```python
from build123d import *

# Parameters (mm, degrees)
F0_W     = 38.1
F0_H     = 38.1
F1_DEPTH = 177.8
F2_T     = -2.54
F3_R     = 2.579688
F4_DEPTH = 355.601
F5_R     = 3.175
F6_DEPTH = 38.101


with BuildPart() as f1:
    # F0 (on Front) → F1 (new body, symmetric)
    with BuildSketch(Plane.XZ):
        Rectangle(F0_W, F0_H)
    extrude(amount=F1_DEPTH, both=True)

    # F2
    f2_openings = [f1.faces().sort_by_distance(p)[0] for p in [
        (-19.05, 0, 0),
        (0, 0, -19.05),
    ]]
    offset(amount=F2_T, openings=f2_openings)

    # F3 (on face) → F4 (cut, through all)
    with BuildSketch(Plane(origin=(0, 177.8, 0), x_dir=(-1, 0, 0), z_dir=(0, 1, 0))):
        Circle(F3_R)
    extrude(amount=-F4_DEPTH, mode=Mode.SUBTRACT)

    # F5 (on face) → F6 (cut, through all)
    with BuildSketch(Plane.YZ.offset(19.05)):
        with Locations((-101.6, 0)):
            Circle(F5_R)
        with Locations((101.6, 0)):
            Circle(F5_R)
    extrude(amount=-F6_DEPTH, mode=Mode.SUBTRACT)


solid = f1.part
```
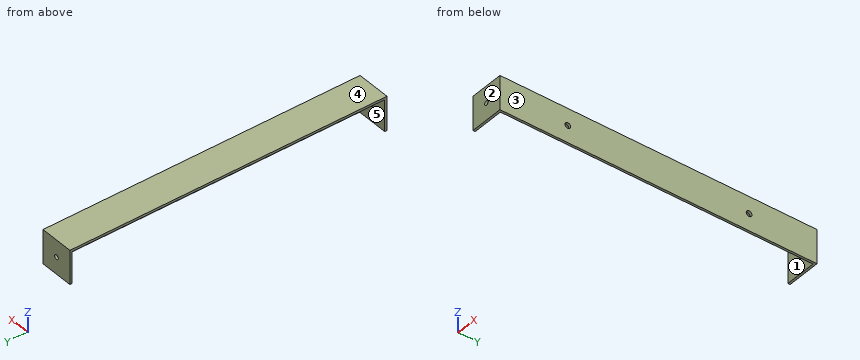
Verification items for the finished model (mm, model axes). Face numbers are marked on the shaded views. A direction names the side the tool comes from. Round coordinates to 2 decimals unless told otherwise and drop trailing zeros. Order: outer loops, then holes, each group sorted by start corner. A loop starts at its lowest first (then second) coordinate and runs counter-clockwise, first axis right, second up. Notation, with made-up numbers: (20.5, 38.5) -> (79.5, 38.5) arc R6 cw to (79.5, 47.5) -> close; hole circle Ø5 at (-17.5, -37). An arc over 180 degrees is marked (long way). Put each result on its own line as item: value. Start each with the question number.
(1) Material ranges on line 1 along Y through (x, z) = (-7.5, -14.5); line 2 along Z through (x, y) = (18.1, 101.6) (3 decimals); line 3 along X through (y, z) = (-80, -16), recorded low to high.
(2) Draft check along Y on the marked faces 1, 2 and 3. Enter one of: +Y half, -Y half, draft (parallel to the pull), parting line (faces both ways), or undercut.
(3) Tool access check on the marked faces 4 and 5. Record the directions out of +Z, -Z, +X, -X, +Y, -Y that give a thin tool (end or side, any length) a straight path to the whole face; none if there is none.
(4) Depth check by flat-ended pin: pin 1 Ø18 at (x, y) = (0.5, 61) entering from -Z; pin 2 Ø8.5 at (x, z) = (0, 0) entering from +Y; pin 3 Ø4 at (x, z) = (0, 0) entering from +Y; pin 4 Ø18 at (y, z) = (20.5, 5) entering from -X. Enter the tip coordinate at first touch or a pass-through.
(5) Section check D-D (y = 8). Enter the section's corners in (x, z), then the cut area to 3 significant figures.
(6) Section check C-C (z = -16). Enter the section's corners in (x, y).
(7) Section check A-A (y = -101.6). Enter the section's corners in (x, z) (3 decimals).
(8) Section check B-B (x = 11). Enter the section's corners in (y, z), then the cut area to 3 significant figures.
Completed:
1. line 1: y = -177.8 to -175.26, 175.26 to 177.8
1. line 2: z = -19.05 to -3.175, 3.175 to 19.05
1. line 3: x = 16.51 to 19.05
2. face 1: undercut
2. face 2: -Y half
2. face 3: draft
3. face 4: +Z, +X, -X, +Y, -Y
3. face 5: -Z, -X
4. pin 1: stops at z = 16.51
4. pin 2: stops at y = 177.8
4. pin 3: passes through
4. pin 4: stops at x = 16.51
5. outline: (-19.05, 16.51) -> (16.51, 16.51) -> (16.51, -19.05) -> (19.05, -19.05) -> (19.05, 19.05) -> (-19.05, 19.05) -> close
5. area: 187 mm2
6. outline: (-19.05, -177.8) -> (19.05, -177.8) -> (19.05, 177.8) -> (-19.05, 177.8) -> (-19.05, 175.26) -> (16.51, 175.26) -> (16.51, -175.26) -> (-19.05, -175.26) -> close
7. outline: (-19.05, 16.51) -> (16.51, 16.51) -> (16.51, 3.175) -> (19.05, 3.175) -> (19.05, 19.05) -> (-19.05, 19.05) -> close; (16.51, -19.05) -> (19.05, -19.05) -> (19.05, -3.175) -> (16.51, -3.175) -> close
8. outline: (-177.8, -19.05) -> (-175.26, -19.05) -> (-175.26, 16.51) -> (175.26, 16.51) -> (175.26, -19.05) -> (177.8, -19.05) -> (177.8, 19.05) -> (-177.8, 19.05) -> close
8. area: 1,080 mm2
